Here's how the part is built. I have some questions about the finished solid (model axes, mm). A direction names the side the tool comes from. Round coordinates to 2 decimals unless told otherwise and drop trailing zeros. Write each loop counter-clockwise with the first axis right and the second up, starting at its lowest first coordinate (ties: lowest second). Pieces come first, ordered by that corner, then holes. Notation, with made-up numbers: (-8, 36) - (0, 36) arc R22 cw to (0, 54) - close; hole circle Ø6 at (17.5, -11). An arc over 180 degrees is marked (long way). Write item = value, one per line. Start each with the question number.
Item 1: Which directions (+Z, -Z, +X, -X, +Y, -Y) give clear straight access to the entire face, cutting with the end or side of a thin tool? Please do faces 1 (the face through (18.058, 2, -18)), 2 (the face through (18.058, 2, -41)), 3 (the face through (-94, 2, 1.475)), 4 (the face through (-94, 2, -33.525)).
Item 2: If we section it at B-B (z = -20): Please give me the cut outline in (x, y), and give its area (3 significant figures).
Item 3: Thinking about a two-plate mould opening in Z: for faces 5 (the face through (21, 2, 1.475)), 6 (the face through (21, 2, -33.525)), 7 (the face through (21, 2, -38.525)), which applies, pulls with the +Z half, pulls with the -Z half, needs draft (parallel to the pull), parting line crosses it, or undercut?
Item 4: If I drill on line 1 along X through (y, z) = (1.6, -17), over which ranges is the centre line in solid material (lowest first)? Write a range as [from, to].
Item 5: For P1, Ø2.5, axis at x = -93.5, y = 1.5, coming from the +Z side; P2, Ø2.5, axis at x = 20.5, y = 1.5, coming from the -Z side; P3, Ø2.5, axis at y = 3, z = -41.5, coming from the -X side, each with a flat end and sliding along its axis, tell me the tip position at first contact or that it passes through.
Item 6: If we section it at A-A (y = 1.4): Please give me the cut outline in (x, z).
```python
from build123d import *

# Parameters (mm, degrees)
SKETCH2_W           = 110
SKETCH2_H           = 50
BOSS_EXTRUDE1_DEPTH = 5
SKETCH3_W           = 5
SKETCH3_H           = 5
BOSS_EXTRUDE2_DEPTH = 5
SKETCH4_W           = 5
SKETCH4_H           = 5
BOSS_EXTRUDE3_DEPTH = 5


with BuildPart() as part:
    # Sketch2 → Boss-Extrude1 (new body)
    with BuildSketch(Plane(origin=(0, 0, 0), x_dir=(1, 0, 0), z_dir=(0, 1, 0))):
        with Locations((-36.942060086, 18.524678112)):
            Rectangle(SKETCH2_W, SKETCH2_H)
    extrude(amount=BOSS_EXTRUDE1_DEPTH)

    # Sketch3 → Boss-Extrude2 (add)
    with BuildSketch(Plane.ZY.offset(91.942060086)):
        with Locations((-36.024678112, 2.5)):
            Rectangle(SKETCH3_W, SKETCH3_H)
        with Locations((-1.024678112, 2.5)):
            Rectangle(SKETCH3_W, SKETCH3_H)
    extrude(amount=BOSS_EXTRUDE2_DEPTH)

    # Sketch4 → Boss-Extrude3 (add)
    with BuildSketch(Plane(origin=(18.057939914, 0, 0), x_dir=(0, 0, -1), z_dir=(1, 0, 0))):
        with Locations((36.024678112, 2.5)):
            Rectangle(SKETCH4_W, SKETCH4_H)
        with Locations((1.024678112, 2.5)):
            Rectangle(SKETCH4_W, SKETCH4_H)
    extrude(amount=BOSS_EXTRUDE3_DEPTH)


solid = part.part
```
Reply:
q1.face_1 = +X, +Y, -Y
q1.face_2 = -Z, +X, +Y, -Y
q1.face_3 = +Z, -X, +Y, -Y
q1.face_4 = -X, +Y, -Y
q2.outline = (-91.94, 0) - (18.06, 0) - (18.06, 5) - (-91.94, 5) - close
q2.area = 550 mm2
q3.face_5 = pulls with the +Z half
q3.face_6 = undercut
q3.face_7 = pulls with the -Z half
q4.line_1 = [-91.94, 18.06]
q5.P1 = 1.48
q5.P2 = -38.52
q5.P3 = -91.94
q6.outline = (-96.94, -38.52) - (-91.94, -38.52) - (-91.94, -43.52) - (18.06, -43.52) - (18.06, -38.52) - (23.06, -38.52) - (23.06, -33.52) - (18.06, -33.52) - (18.06, -3.52) - (23.06, -3.52) - (23.06, 1.48) - (18.06, 1.48) - (18.06, 6.48) - (-91.94, 6.48) - (-91.94, 1.48) - (-96.94, 1.48) - (-96.94, -3.52) - (-91.94, -3.52) - (-91.94, -33.52) - (-96.94, -33.52) - close
